Check sheet for the drawn part. Datum: minimum x, y, z corner. Units: mm. A direction names the side the tool comes from. Give positions to 0.01 mm unless a question says otherwise; leave off trailing zeros. Order: outer loops, then holes, each group sorted by start corner. A loop starts at its lowest first (then second) coordinate and runs counter-clockwise, first axis right, second up. Notation, with made-up numbers: (35.5, 83.25) -> (66.5, 83.25) arc R26 cw to (66.5, 103.25) -> close; hole circle Ø1 at (49.25, -11). An arc over 180 degrees is marked (long way). Return JSON: item names as keys, results as strings. Group by question number.
(1) Tool access check on the marked faces 1 and 2. Record the directions out of +Z, -Z, +X, -X, +Y, -Y that give a thin tool (end or side, any length) a straight path to the whole face; none if there is none.
(2) Release check for a two-part mould opening along X. For the marked faces 3, 4 and 5 record: pulls with the +X half, pulls with the -X half, needs draft (parallel to the pull), parting line crosses it, or undercut.
(3) Cross-section at B-B on y = 30. Enter the section's corners in (x, z), then the cut area to 3 significant figures.
(4) Cross-section at D-D on y = 13. Enter the section's corners in (x, z), then the cut area to 3 significant figures.
(5) Cross-section at A-A on x = 55. Enter the section's corners in (y, z), then the cut area to 3 significant figures.
(6) Cross-section at C-C on z = 33.5. Enter the section's corners in (x, y).
(7) Depth check by flat-ended pin: pin 1 Ø12 at (x, y) = (77.5, 35) entering from +Z. Enter the tip coordinate at first touch or a pass-through.
(8) Thickness scan on line 1 along X through (y, z) = (18, 60); line 2 along Y through (x, z) = (55, 12); line 3 along Z through (x, y) = (66, 9.5). Record the ranges inside material, lowest first.
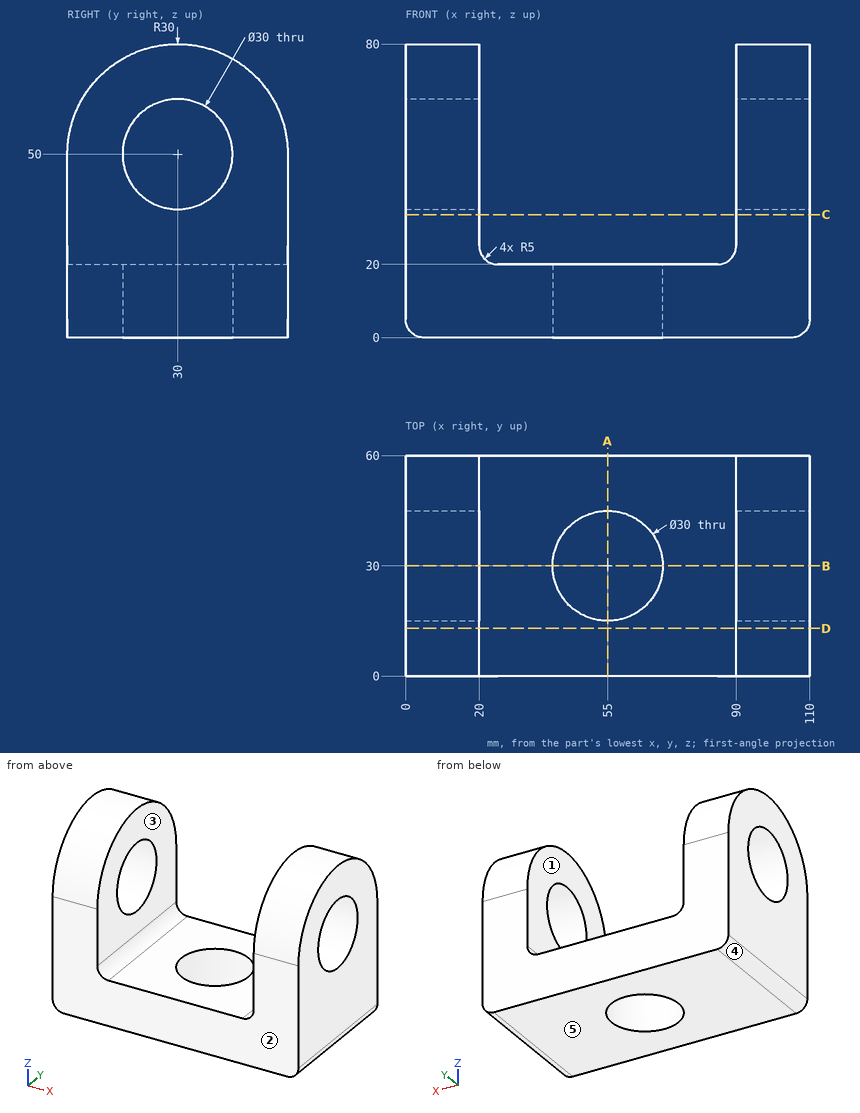
Verdict:
{
 "1": {"face 1": "+Z, +Y, -Y", "face 2": "+Z, -Z, +X, -X, -Y"},
 "2": {"face 3": "undercut", "face 4": "pulls with the -X half", "face 5": "needs draft"},
 "3": {"outline": "(0, 5) arc R5 ccw to (5, 0) -> (40, 0) -> (40, 20) -> (25, 20) arc R5 cw to (20, 25) -> (20, 35) -> (0, 35) -> close; (0, 65) -> (20, 65) -> (20, 80) -> (0, 80) -> close; (70, 0) -> (105, 0) arc R5 ccw to (110, 5) -> (110, 35) -> (90, 35) -> (90, 25) arc R5 cw to (85, 20) -> (70, 20) -> close; (90, 65) -> (110, 65) -> (110, 80) -> (90, 80) -> close", "area": "2,800 mm²"},
 "4": {"outline": "(0, 5) arc R5 ccw to (5, 0) -> (105, 0) arc R5 ccw to (110, 5) -> (110, 74.72) -> (90, 74.72) -> (90, 25) arc R5 cw to (85, 20) -> (25, 20) arc R5 cw to (20, 25) -> (20, 74.72) -> (0, 74.72) -> close", "area": "4,390 mm²"},
 "5": {"outline": "(0, 0) -> (15, 0) -> (15, 20) -> (0, 20) -> close; (45, 0) -> (60, 0) -> (60, 20) -> (45, 20) -> close", "area": "600 mm²"},
 "6": {"outline": "(0, 0) -> (20, 0) -> (20, 60) -> (0, 60) -> close; (90, 0) -> (110, 0) -> (110, 60) -> (90, 60) -> close"},
 "7": {"pin 1": "z = 20"},
 "8": {"line 1": "0 to 20, 90 to 110", "line 2": "0 to 15, 45 to 60", "line 3": "0 to 20"}
}
